Build history of the part. All positions in model axes, mm. Face numbers are marked on the shaded views. A direction names the side the tool comes from. Give positions to 0.01 mm unless a question says otherwise; leave off trailing zeros. Order: outer loops, then holes, each group sorted by start corner. A loop starts at its lowest first (then second) coordinate and runs counter-clockwise, first axis right, second up. Notation, with made-up numbers: M 50,-8.75 L 88,-8.75 A12 ccw 88,-3.75 Z; hole C -23,51.5 d5. An arc over 180 degrees is marked long. Answer as CSV lines item,"result".
from build123d import *

# Parameters (mm, degrees)
F0_R     = 18.45
F0_R_2   = 6.9
F1_DEPTH = 3.2
F2_R     = 8.75
F2_R_2   = 6.9
F3_DEPTH = 5
F4_SIZE  = 0.5
F5_SIZE  = 0.2


with BuildPart() as f1:
    # F0 (on Top) → F1 (new body)
    with BuildSketch(Plane.XY):
        Circle(F0_R)
        Circle(F0_R_2, mode=Mode.SUBTRACT)
    extrude(amount=F1_DEPTH)

    # F2 (on face) → F3 (join)
    with BuildSketch(Plane.XY.offset(3.2)):
        Circle(F2_R)
        Circle(F2_R_2, mode=Mode.SUBTRACT)
    extrude(amount=F3_DEPTH)

    # F4
    f4_edges = [f1.edges().sort_by_distance(p)[0] for p in [
        (-18.45, 0, 0),
    ]]
    chamfer(f4_edges, length=F4_SIZE)

    # F5
    f5_edges = [f1.edges().sort_by_distance(p)[0] for p in [
        (-6.9, 0, 0),
        (-6.9, 0, 8.2),
        (-8.75, 0, 8.2),
        (-8.75, 0, 3.2),
        (-18.45, 0, 3.2),
    ]]
    chamfer(f5_edges, length=F5_SIZE)


solid = f1.part
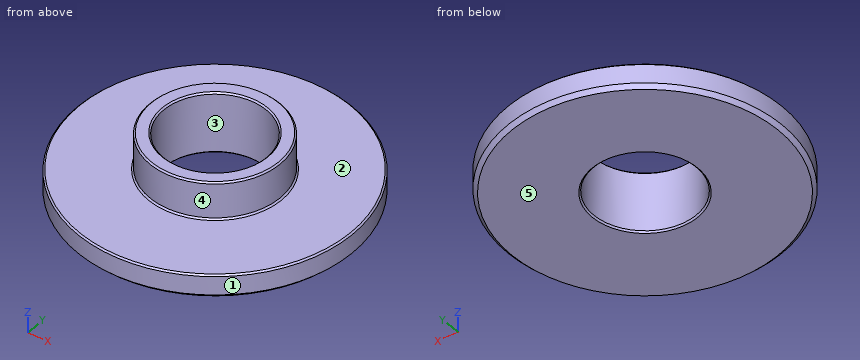
Item 1: Drop flat-ended pins along their axis: pin 1 (1 mm diameter, centred on x = -2.5, z = 7.5, fed in from +Y); pin 2 (3 mm diameter, centred on x = 13, y = 12.5, fed in from -Z); pin 3 (4 mm diameter, centred on y = 4.5, z = 7.5, fed in from -X); pin 4 (1.5 mm diameter, centred on y = 7, z = 2, fed in from +X). Give the stop position or say it passes through.
Geometry says:
pin 1,"stops at y = 8.52"
pin 2,"stops at z = 0"
pin 3,"stops at x = -8.39"
pin 4,"stops at x = 17.36"
Item 2: Band-saw the part on D-D (z = 1.25). Give the cut face in (x, y), and give its area (3 significant figures).
Geometry says:
outline,"C 0,0 d36.9; hole C 0,0 d13.8"
area,"920 mm2"
Item 3: Band-saw the part on C-C (z = 7). Give the cut face in (x, y).
Geometry says:
outline,"C 0,0 d17.5; hole C 0,0 d13.8"
Item 4: Probe line 1 along Y through (x, z) = (0, 4.25); line 2 along Z through (x, y) = (-8.5, -1); line 3 along Z through (x, y) = (10.5, 6). List the from-to ranges inside material, lowest first. Write a range as from..to.
Geometry says:
line 1,"y = -8.75..-6.9, 6.9..8.75"
line 2,"z = 0..8.19"
line 3,"z = 0..3.2"
Item 5: 3-axis set-ups, long thin cutter, end or side, ignore diameter. For the marked faces 4 and 5: which of +Z, -Z, +X, -X, +Y, -Y reach the whole face in a straight line?
Geometry says:
face 4,"+Z"
face 5,"-Z, +X, -X, +Y, -Y"
Item 6: Pull direction Y, two halves, no side cores. Call the marked faces 1, 2 and 3: released by +Y, released by -Y, zero draft, split by the parting line, or undercut.
Geometry says:
face 1,"split by the parting line"
face 2,"zero draft"
face 3,"undercut"
Item 7: Band-saw the part on A-A (y = 0). Give the cut face in (x, z).
Geometry says:
outline,"M -18.45,0.5 L -17.95,0 L -7.1,0 L -6.9,0.2 L -6.9,8 L -7.1,8.2 L -8.55,8.2 L -8.75,8 L -8.75,3.4 L -8.95,3.2 L -18.25,3.2 L -18.45,3 Z; M 6.9,0.2 L 7.1,0 L 17.95,0 L 18.45,0.5 L 18.45,3 L 18.25,3.2 L 8.95,3.2 L 8.75,3.4 L 8.75,8 L 8.55,8.2 L 7.1,8.2 L 6.9,8 Z"
